```python
from build123d import *

# Parameters (mm, degrees)
F1_DEPTH = 4
F0_W     = 23
F0_H     = 4
F0_W_2   = 15
F0_H_2   = 1
F2_DEPTH = 23
F3_R     = 9.5
F4_DEPTH = 25
F5_R     = 5
F6_R     = 5
F7_R     = 0.75


with BuildPart() as f1:
    # F0 (on Top) → F1 (new body)
    with BuildSketch(Plane.XY):
        Polygon((-8.587917, 10.685558), (-11.587917, 10.685558), (-11.587917, -21.314442), (-8.587917, -21.314442), (-8.587917, -19.314442), (-8.587917, -12.314442), (-8.587917, 3.685558), align=None)
        with BuildLine():
            Line((-0.587917, -12.314442), (-8.587917, -12.314442))
            Line((-8.587917, -12.314442), (-8.587917, -19.314442))
            Line((-8.587917, -19.314442), (-0.587917, -19.314442))
            Line((-0.587917, -19.314442), (-0.587917, -17.560003))
            Line((-0.587917, -17.560003), (-4.463338, -17.560003))
            ThreePointArc((-4.463338, -17.560003), (-4.587917, -17.564442), (-4.712495, -17.560003))
            ThreePointArc((-4.712495, -17.560003), (-6.336806, -15.752114), (-4.587917, -14.064442))
            Line((-4.587917, -14.064442), (-0.587917, -14.064442))
            Line((-0.587917, -14.064442), (-0.587917, -12.314442))
        make_face()
        with BuildLine():
            Line((-0.587917, 10.685558), (-8.587917, 10.685558))
            Line((-8.587917, 10.685558), (-8.587917, 3.685558))
            Line((-8.587917, 3.685558), (-0.587917, 3.685558))
            Line((-0.587917, 3.685558), (-0.587917, 5.436083))
            Line((-0.587917, 5.436083), (-4.545018, 5.436083))
            ThreePointArc((-4.545018, 5.436083), (-4.587917, 5.435558), (-4.630815, 5.436083))
            ThreePointArc((-4.630815, 5.436083), (-6.337785, 7.207009), (-4.587917, 8.935558))
            Line((-4.587917, 8.935558), (-0.587917, 8.935558))
            Line((-0.587917, 8.935558), (-0.587917, 10.685558))
        make_face()
        Polygon((-8.587917, -21.314442), (-11.587917, -21.314442), (-25.587917, -21.314442), (-25.587917, -25.314442), (-8.587917, -25.314442), align=None)
    extrude(amount=F1_DEPTH)

    # F0 (on Top) → F2 (join)
    with BuildSketch(Plane.XY):
        with Locations((-37.087917, -23.314442)):
            Rectangle(F0_W, F0_H)
        with Locations((-37.087917, -23.314442)):
            Rectangle(F0_W_2, F0_H_2, mode=Mode.SUBTRACT)
        with Locations((-37.087917, -23.314442)):
            Rectangle(F0_W_2, F0_H_2)
    extrude(amount=F2_DEPTH)

    # F3 (on face) → F4 (cut)
    with BuildSketch(Plane.XZ.offset(25.314442)):
        with Locations((-37.087917, 11.5)):
            Circle(F3_R)
    extrude(amount=-F4_DEPTH, mode=Mode.SUBTRACT)

    # F5
    f5_edges = [f1.edges().sort_by_distance(p)[0] for p in [
        (-48.587917, -23.314442, 23),
        (-25.587917, -23.314442, 23),
        (-48.587917, -23.314442, 0),
        (-25.587917, -23.314442, 4),
    ]]
    fillet(f5_edges, radius=F5_R)

    # F6
    f6_edges = [f1.edges().sort_by_distance(p)[0] for p in [
        (-8.587917, -25.314442, 2),
        (-11.587917, -21.314442, 2),
        (-8.587917, -12.314442, 2),
        (-8.587917, 3.685558, 2),
        (-11.587917, 10.685558, 2),
    ]]
    fillet(f6_edges, radius=F6_R)

    # F7
    f7_edges = [f1.edges().sort_by_distance(p)[0] for p in [
        (-0.587917, 10.685558, 2),
        (-0.587917, 8.935558, 2),
        (-0.587917, 5.436083, 2),
        (-0.587917, 3.685558, 2),
        (-0.587917, -12.314442, 2),
        (-0.587917, -14.064442, 2),
        (-0.587917, -17.560003, 2),
        (-0.587917, -19.314442, 2),
    ]]
    fillet(f7_edges, radius=F7_R)


solid = f1.part
```
Model file for the job. Use its own axes, mm. A direction names the side the tool comes from. Round coordinates to 2 decimals unless told otherwise and drop trailing zeros. Loops run counter-clockwise (first coordinate to the right, second up) from the corner with the lowest first, then second, coordinate; pieces in that order, holes last. Notation, with made-up numbers: M 0.25,6 L 40.25,6 A27 cw 40.25,28 Z; hole C 54.5,14 d11. An arc over 180 degrees is marked long. Put each result on its own line as item: value. Start each with the question number.
Item 1: Drop flat-ended pins along their axis: P1, Ø5, axis at x = -11, z = 3.5, coming from the +Y side; P2, Ø3.5, axis at x = -2.5, z = 2, coming from the -Y side; P3, Ø0.8, axis at y = -20, z = 2, coming from the +X side; P4, Ø12, axis at y = -14, z = 15, coming from the +X side. Give the stop position or say it passes through.
Item 2: Cut at B-B (x = -29). List the corners of the cut face in (y, z).
Item 3: Mould opens along Y. For faces 4 (the face through (-4, 10.686, 2)), 5 (the face through (-7.084, -10.889, 2.028)), 6 (the face through (-5, -19.314, 2)) say: released by +Y, released by -Y, zero draft, split by the parting line, or undercut.
Item 4: 3-axis set-ups, long thin cutter, end or side, ignore diameter. For faces 1 (the face through (-3, 5.436, 2)), 2 (the face through (-25.588, -23, 13)), 3 (the face through (-29, -21.314, 4)): which of +Z, -Z, +X, -X, +Y, -Y reach the whole face in a straight line?
Item 5: Drill centre lines: line 1 along Z through (x, y) = (-11.5, -16); line 2 along X through (y, z) = (-23, 15); line 3 along X through (y, z) = (4.5, 3.75). Where is each one in solid material? Low to high.
Item 6: Cut at C-C (y = -23). List the corners of the cut face in (x, z), then the cut area to 3 significant figures.
Item 7: Cut at D-D (y = -9.5). List the corners of the cut face in (x, z).
Item 8: Cut at A-A (z = 11.5). List the corners of the cut face in (x, y).
Answer block:
1. P1: y = 10.31
1. P2: y = -19.31
1. P3: x = -8.59
1. P4: through
2. outline: M -25.31,0 L -21.31,0 L -21.31,6.52 L -25.31,6.52 Z; M -25.31,16.48 L -21.31,16.48 L -21.31,22.74 L -25.31,22.74 Z
3. face 4: released by +Y
3. face 5: undercut
3. face 6: released by -Y
4. face 1: +Z, -Z, +X
4. face 2: +Z, +X, +Y, -Y
4. face 3: +Z, -Z, -X, +Y
5. line 1: 0 to 4
5. line 2: -48.59 to -45.92, -28.26 to -25.59
5. line 3: -11.59 to -0.59
6. outline: M -48.59,5 A5 ccw -43.59,0 L -9.37,0 L -9.37,4 L -20.59,4 A5 cw -25.59,9 L -25.59,18 A5 ccw -30.59,23 L -43.59,23 A5 ccw -48.59,18 Z; hole C -37.09,11.5 d19
6. area: 300 mm2
7. outline: M -11.59,0 L -8.08,0 L -8.08,4 L -11.59,4 Z
8. outline: M -48.59,-25.31 L -46.59,-25.31 L -46.59,-21.31 L -48.59,-21.31 Z; M -27.59,-25.31 L -25.59,-25.31 L -25.59,-21.31 L -27.59,-21.31 Z
